Source: CAD feature listing. Evaluate the final solid. Frame: model axes, mm. A direction names the side the tool comes from. Coordinates: 2 decimals unless noted, no trailing zeros. Loops run counter-clockwise (first coordinate to the right, second up) from the corner with the lowest first, then second, coordinate; pieces in that order, holes last. Notation, with made-up numbers: (21, 70.5) -> (51, 70.5) arc R13 ccw to (51, 81.5) -> close; hole circle Ø5 at (-2, 86). An arc over 180 degrees is marked (long way). Answer as CSV lines item,"result".
from build123d import *

# Parameters (mm, degrees)
SKETCH1_W           = 40
SKETCH1_H           = 120
SKETCH1_R           = 7.5
BOSS_EXTRUDE1_DEPTH = 30
FILLET1_R           = 15
SKETCH2_R           = 7.5
CUT_EXTRUDE1_DEPTH  = 15
FILLET2_R           = 15


with BuildPart() as part:
    # Sketch1 → Boss-Extrude1 (new body)
    with BuildSketch(Plane(origin=(0, 0, 0), x_dir=(0, 0, -1), z_dir=(1, 0, 0))):
        Rectangle(SKETCH1_W, SKETCH1_H)
        with Locations((0, 40)):
            Circle(SKETCH1_R, mode=Mode.SUBTRACT)
        with Locations((0, -40)):
            Circle(SKETCH1_R, mode=Mode.SUBTRACT)
    extrude(amount=BOSS_EXTRUDE1_DEPTH)

    # Fillet1
    fillet1_edges = [part.edges().sort_by_distance(p)[0] for p in [
        (15, 60, 20),
        (15, 60, -20),
        (15, -60, -20),
        (15, -60, 20),
    ]]
    fillet(fillet1_edges, radius=FILLET1_R)

    # Sketch2 → Cut-Extrude1 (cut)
    with BuildSketch(Plane(origin=(30, 0, 0), x_dir=(0, 0, -1), z_dir=(1, 0, 0))):
        with BuildLine():
            Line((-20, 45), (-20, 15))
            Line((-20, 15), (20, 15))
            Line((20, 15), (20, 45))
            ThreePointArc((20, 45), (15.606601718, 55.606601718), (5, 60))
            Line((5, 60), (-5, 60))
            ThreePointArc((-5, 60), (-15.606601718, 55.606601718), (-20, 45))
        make_face()
        with Locations((0, 40)):
            Circle(SKETCH2_R, mode=Mode.SUBTRACT)
    extrude(amount=-CUT_EXTRUDE1_DEPTH, mode=Mode.SUBTRACT)

    # Fillet2
    fillet2_edges = [part.edges().sort_by_distance(p)[0] for p in [
        (22.5, 15, 20),
        (22.5, 15, -20),
    ]]
    fillet(fillet2_edges, radius=FILLET2_R)


solid = part.part
(1) Pin query (flat end, axial travel): pin 1 Ø6 at (x, z) = (19.5, -12.5) entering from -Y; pin 2 Ø10 at (x, z) = (9, -12) entering from -Y; pin 3 Ø8 at (x, z) = (20, 1.5) entering from +Y; pin 4 Ø9 at (y, z) = (40, 0) entering from -X. Return the tip coordinate at first contact, or that it passes through.
Computed values:
pin 1,"y = -59.31"
pin 2,"y = -59.87"
pin 3,"y = 15"
pin 4,"through"
(2) Cut plane B-B (z = 0). Return the cut outline in (x, y), then the cut area to 3 significant figures.
Computed values:
outline,"(0, -60) -> (30, -60) -> (30, -47.5) -> (0, -47.5) -> close; (0, -32.5) -> (30, -32.5) -> (30, 15) -> (15, 15) -> (15, 32.5) -> (0, 32.5) -> close; (0, 47.5) -> (15, 47.5) -> (15, 60) -> (0, 60) -> close"
area,"2,250 mm^2"
(3) Cut plane D-D (y = 40). Return the cut outline in (x, z), then the cut area to 3 significant figures.
Computed values:
outline,"(0, -20) -> (15, -20) -> (15, -7.5) -> (0, -7.5) -> close; (0, 7.5) -> (15, 7.5) -> (15, 20) -> (0, 20) -> close"
area,"375 mm^2"
(4) Draft query along Z for faces 1 (the cylindrical face through (7.4, 32.68, 1.63)), 2 (the flat face through (0, 1, 0)), 3 (the flat face through (11, -11, 20)), 4 (the cylindrical face through (14.79, -47.32, 1.63)). Return one class per face: released by +Z, released by -Z, zero draft, split by the parting line, or undercut.
Computed values:
face 1,"undercut"
face 2,"zero draft"
face 3,"released by +Z"
face 4,"undercut"
(5) Cut plane A-A (y = -40). Return the cut outline in (x, z).
Computed values:
outline,"(0, -20) -> (30, -20) -> (30, -7.5) -> (0, -7.5) -> close; (0, 7.5) -> (30, 7.5) -> (30, 20) -> (0, 20) -> close"
(6) Material intervals for L1, parallel to Y at x = 5.75, z = 0; L2, parallel to Y at x = 22.75, z = 0; L3, parallel to X at y = 27.5, z = 1.5, sorted ascending. Write a range as [from, to].
Computed values:
L1,"[-60, -47.5], [-32.5, 32.5], [47.5, 60]"
L2,"[-60, -47.5], [-32.5, 15]"
L3,"[0, 15]"
(7) Access query for faces 5 (the cylindrical face through (22.4, 10.49, 15.72)), 6 (the flat face through (23, 15, 0)), 7 (the cylindrical face through (22.4, 10.72, -15.49)). Directions: +Z, -Z, +X, -X, +Y, -Y. A direction counts if a zero-diameter tool reaches every point of the face in a straight line with its end or side. Return the directions, or none.
Computed values:
face 5,"+Z, +X, +Y"
face 6,"+Z, -Z, +X, +Y"
face 7,"-Z, +X, +Y"
(8) Cut plane C-C (x = 16.75). Return the cut outline in (y, z), then the cut area to 3 significant figures.
Computed values:
outline,"(-60, -5) arc R15 ccw to (-45, -20) -> (0, -20) arc R15 ccw to (15, -5) -> (15, 5) arc R15 ccw to (0, 20) -> (-45, 20) arc R15 ccw to (-60, 5) -> close; hole circle Ø15 at (-40, 0)"
area,"2,630 mm^2"
